Autodesk Inventor part; units mm, degrees
ref_plane "YZ Plane" through (0, 0, 0) normal (1, 0, 0) x (0, 1, 0)
ref_plane "XZ Plane" through (0, 0, 0) normal (0, 1, 0) x (-1, 0, 0)
ref_plane "XY Plane" through (0, 0, 0) normal (0, 0, 1) x (1, 0, 0)
sketch "Sketch1" plane through (0, 0, 0) normal (0, 1, 0) x (-1, 0, 0)
  circle A0 centre (0, 0) radius 63.5
  dimension "d0" = 127
extrude "Extrusion1" add sketch "Sketch1" along normal blind 10
sketch "Sketch2" plane through (0, 10, 0) normal (0, 1, 0) x (1, 0, 0)
  line L0 (0, 0) -> (0, 63.7295)
  circle A0 centre (0, 0) radius 63.5
  line L1 (7.5, 44.1365) -> (-7.5, 44.1365)
  line L2 (-7.5, 44.1365) -> (-7.5, 64.1365)
  line L3 (-7.5, 64.1365) -> (7.5, 64.1365)
  line L4 (7.5, 64.1365) -> (7.5, 44.1365)
  line L5 (7.5, 44.1365) -> (-7.5, 64.1365) construction
  line L6 (-7.5, 44.1365) -> (7.5, 64.1365) construction
  point P0 (0, 54.1365)
  point P1 (-7.5, 63.0555)
  point P2 (7.5, 63.0555)
  dimension "d3" = 15
  dimension "d4" = 20
extrude "Extrusion2" add sketch "Sketch2" along normal blind 15 contours L1 L2 A0 L0 | L0 A0 L4 L1
pattern_circular "Circular Pattern1" count 3 over 360 about axis through (0, 0, 0) along (0, 1, 0) of "Extrusion2"
sketch "Sketch3" plane through (0, 0, 0) normal (0, -1, 0) x (1, 0, 0)
  circle A0 centre (0, 0) radius 15
  dimension "d10" = 30
extrude "Extrusion3" add sketch "Sketch3" along normal blind 5
properties part number "PM Base"
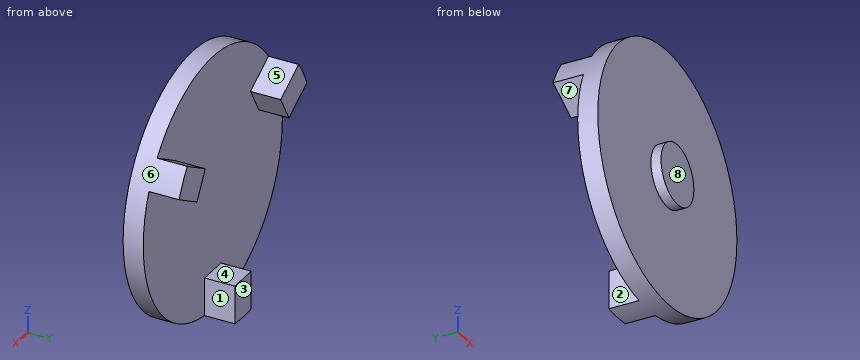
Here's how the part is built. I have some questions about the finished solid (model axes, mm). Face numbers are marked on the shaded views. A direction names the side the tool comes from. Coordinates: 2 decimals unless noted, no trailing zeros. Order: outer loops, then holes, each group sorted by start corner. A loop starts at its lowest first (then second) coordinate and runs counter-clockwise, first axis right, second up. Notation, with made-up numbers: (0, 70) - (7, 70) arc R33 ccw to (7, 108) - close; hole circle Ø11 at (-9, 44). An arc over 180 degrees is marked (long way). One line per question, with ' | ' between items. Start each with the question number.
1. Which directions (+Z, -Z, +X, -X, +Y, -Y) give clear straight access to the entire face, cutting with the end or side of a thin tool? Please do the marked faces 1, 2, 3 and 4.
2. If we section it at B-B (z = 0): Write out the boundary of the cut face in (x, y).
3. If we section it at A-A (y = 11.5): Write out the boundary of the cut face in (x, z), and give its area (3 significant figures).
4. If we section it at D-D (y = 1.5): Write out the boundary of the cut face in (x, z), and give its area (3 significant figures).
5. Please list where these lines run through material, in increasing order: line 1 along Y through (x, z) = (-12, 53); line 2 along Y through (x, z) = (-3.5, -52); line 3 along X through (y, z) = (14.5, 30). Write a range as [from, to].
6. I'm going to push flat-ended pins straight in: pin 1 Ø12 at (x, y) = (16, 15.5) entering from +Z; pin 2 Ø7.5 at (x, y) = (-3, 16) entering from +Z; pin 3 Ø5 at (x, y) = (-43.5, 4.5) entering from +Z. Where does each tip first touch, or does it pass through?
7. If we mould it in two halves opening along X, with no side actions, what happens to the marked faces 5, 6, 7 and 8? For each: released by +X, released by -X, zero draft, split by the parting line, or undercut.
8. If we section it at C-C (x = 0): Write out the boundary of the cut face in (y, z), and give its area (3 significant figures).
Model answer:
1) face 1: +Z, -Z, +X, +Y | face 2: +Z, -Z, -X, +Y | face 3: +Z, -Z, +X, -X, +Y | face 4: +Z, +X, -X, +Y
2) outline: (-63.5, 0) - (-15, 0) - (-15, -5) - (15, -5) - (15, 0) - (63.5, 0) - (63.5, 10) - (-63.5, 10) - close
3) outline: (-58.36, 25.03) - (-41.97, 15.57) - (-34.47, 28.56) - (-50.86, 38.02) arc R63.5 ccw to start; (-7.5, -63.06) arc R63.5 ccw to (7.5, -63.06) - (7.5, -44.14) - (-7.5, -44.14) - close; (34.47, 28.56) - (41.97, 15.57) - (58.36, 25.03) arc R63.5 ccw to (50.86, 38.02) - close | area: 865 mm²
4) outline: circle Ø127 at (0, 0) | area: 12,700 mm²
5) line 1: y = [0, 10] | line 2: y = [0, 25] | line 3: x = [-55.97, -36.96], [36.96, 55.97]
6) pin 1: stops at z = 62.03 | pin 2: stops at z = -44.14 | pin 3: stops at z = 48.49
7) face 5: undercut | face 6: split by the parting line | face 7: released by -X | face 8: zero draft
8) outline: (-5, -15) - (0, -15) - (0, -63.5) - (25, -63.5) - (25, -44.14) - (10, -44.14) - (10, 63.5) - (0, 63.5) - (0, 15) - (-5, 15) - close | area: 1,710 mm²
